Geometry check sheet. Reference: the model listing, model coordinates, mm. A direction names the side the tool comes from. Round coordinates to 2 decimals unless told otherwise and drop trailing zeros. Order: outer loops, then holes, each group sorted by start corner. A loop starts at its lowest first (then second) coordinate and runs counter-clockwise, first axis right, second up. Notation, with made-up numbers: (59.25, -34) - (105.25, -34) arc R25 cw to (105.25, -10) - close; hole circle Ø7 at (3.5, 65). An arc over 180 degrees is marked (long way). Use a Markdown table: item, result. Add a question column.
(1) Section check B-B on x = 0. Record the boundary of the cut face in (y, z) (3 decimals).
(2) Gauge pin test, flat ends, axial feed: P1, Ø1, axis at x = -1.5, z = -19, coming from the +Y side; P2, Ø19.5, axis at x = 5, z = 8.5, coming from the +Y side. Record the tip position at first contact, or that the pin passes through.
(3) Access from +Z, -Z, +X, -X, +Y, -Y to the whole of each face (thin tool, end or side, straight path). Record for faces 4 (the face through (0, 9, -25.4)), 5 (the face through (3.175, 6, 22)), 6 (the face through (3, 12.7, -6)).
(4) Section check D-D on z = 0. Record the boundary of the cut face in (x, y) (3 decimals), then the cut area to 3 significant figures.
(5) Section check C-C on y = 31. Record the boundary of the cut face in (x, z), then the cut area to 3 significant figures.
(6) Thickness scan on line 1 along Y through (x, z) = (-17.25, -12.7); line 2 along X through (y, z) = (44, 0); line 3 along Z through (x, y) = (-21, 57). Record the ranges inside material, lowest first. Write a range as [from, to].
(7) Mould release check, pull along Z, two halves, no side actions. Record for faces 1 (the face through (14.29, 13.61, 0.36)), 2 (the face through (14, 6, 25.4)), 3 (the face through (-3.86, 6.44, -5.04)): released by +Z, released by -Z, zero draft, split by the parting line, or undercut.
(8) Section check A-A on z = -12.7. Record the boundary of the cut face in (x, y) (3 decimals).
```python
from build123d import *

# Parameters (mm, degrees)
SKETCH1_W           = 50.8
SKETCH1_H           = 50.8
BOSS_EXTRUDE1_DEPTH = 12.7
SKETCH2_R           = 6.1
BOSS_EXTRUDE2_DEPTH = 10.16
SKETCH3_R           = 6.35
CUT_EXTRUDE1_DEPTH  = 68.501425911
FILLET1_R           = 3.175


with BuildPart() as part:
    # Sketch1 → Boss-Extrude1 (new body)
    with BuildSketch(Plane(origin=(0, 0, 0), x_dir=(1, 0, 0), z_dir=(0, 1, 0))):
        Rectangle(SKETCH1_W, SKETCH1_H)
    extrude(amount=BOSS_EXTRUDE1_DEPTH)

    # Sketch2 → Boss-Extrude2 (add)
    with BuildSketch(Plane(origin=(25.4, 0, 0), x_dir=(0, 0, -1), z_dir=(1, 0, 0))):
        with BuildLine():
            Line((-25.4, 0), (-25.4, 12.7))
            Line((-25.4, 12.7), (1.494117647, 63.126470588))
            ThreePointArc((1.494117647, 63.126470588), (15.780202438, 69.470809752), (25.4, 57.15))
            Line((25.4, 57.15), (25.4, 0))
            Line((25.4, 0), (-25.4, 0))
        make_face()
        with Locations((12.7, 57.15)):
            Circle(SKETCH2_R, mode=Mode.SUBTRACT)
    boss_extrude2 = extrude(amount=-BOSS_EXTRUDE2_DEPTH)

    # Mirror1: Boss-Extrude2 across plane
    add(boss_extrude2.mirror(Plane(origin=(0, 0, 0), x_dir=(0, 0, 1), z_dir=(1, 0, 0))))

    # Sketch3 → Cut-Extrude1 (cut, through all)
    with BuildSketch(Plane(origin=(0, 12.7, 0), x_dir=(1, 0, 0), z_dir=(0, 1, 0))):
        with Locations(Location((0, 0, 0), (0, 0, 270))):
            Circle(SKETCH3_R)
        with BuildLine():
            Line((-3.175, -25.4), (-3.175, -19.05))
            ThreePointArc((-3.175, -19.05), (0, -15.875), (3.175, -19.05))
            Line((3.175, -19.05), (3.175, -25.4))
            Line((3.175, -25.4), (-3.175, -25.4))
        make_face()
    extrude(amount=-CUT_EXTRUDE1_DEPTH, mode=Mode.SUBTRACT)

    # Fillet1
    fillet1_edges = [part.edges().sort_by_distance(p)[0] for p in [
        (15.24, 12.7, 0),
        (-15.24, 12.7, 0),
    ]]
    fillet(fillet1_edges, radius=FILLET1_R)


solid = part.part
```
Check sheet entries:
| question | item | result |
|---|---|---|
| 1 | outline | (0, -25.4) - (12.7, -25.4) - (12.7, -6.35) - (0, -6.35) - close; (0, 6.35) - (12.7, 6.35) - (12.7, 15.875) - (0, 15.875) - close |
| 2 | P1 | stops at y = 12.7 |
| 2 | P2 | stops at y = 14.18 |
| 3 | face 4 | -Z, +X, -X, +Y, -Y |
| 3 | face 5 | +Z, +Y, -Y |
| 3 | face 6 | +Z, -Z, +Y |
| 4 | outline | (-25.4, 0) - (-6.35, 0) - (-6.35, 12.7) - (-12.065, 12.7) arc R3.175 cw to (-15.24, 15.875) - (-15.24, 60.325) - (-25.4, 60.325) - close; (6.35, 0) - (25.4, 0) - (25.4, 60.325) - (15.24, 60.325) - (15.24, 15.875) arc R3.175 cw to (12.065, 12.7) - (6.35, 12.7) - close |
| 4 | area | 1,460 mm2 |
| 5 | outline | (-25.4, -25.4) - (-15.24, -25.4) - (-15.24, 15.64) - (-25.4, 15.64) - close; (15.24, -25.4) - (25.4, -25.4) - (25.4, 15.64) - (15.24, 15.64) - close |
| 5 | area | 834 mm2 |
| 6 | line 1 | y = [0, 51.05], [63.25, 69.85] |
| 6 | line 2 | x = [-25.4, -15.24], [15.24, 25.4] |
| 6 | line 3 | z = [-25.4, -18.8], [-6.6, 1.77] |
| 7 | face 1 | zero draft |
| 7 | face 2 | released by +Z |
| 7 | face 3 | undercut |
| 8 | outline | (-25.4, 0) - (25.4, 0) - (25.4, 51.05) - (15.24, 51.05) - (15.24, 15.875) arc R3.175 cw to (12.065, 12.7) - (-12.065, 12.7) arc R3.175 cw to (-15.24, 15.875) - (-15.24, 51.05) - (-25.4, 51.05) - close; (-25.4, 63.25) - (-15.24, 63.25) - (-15.24, 69.85) - (-25.4, 69.85) - close; (15.24, 63.25) - (25.4, 63.25) - (25.4, 69.85) - (15.24, 69.85) - close |
